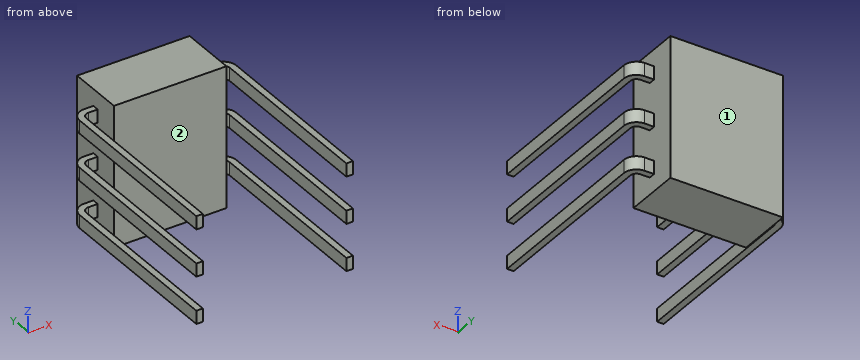
Autodesk Inventor part; units mm, degrees
ref_plane "YZ Plane" through (0, 0, 0) normal (1, 0, 0) x (0, 1, 0)
ref_plane "XZ Plane" through (0, 0, 0) normal (0, 1, 0) x (-1, 0, 0)
ref_plane "XY Plane" through (0, 0, 0) normal (0, 0, 1) x (1, 0, 0)
sketch "Sketch2" plane through (0, 0, 0) normal (0, 0, 1) x (1, 0, 0)
  line L0 (3, -1.5) -> (-3, -1.5)
  line L1 (-3, -1.5) -> (-3, 1.5)
  line L2 (-3, 1.5) -> (3, 1.5)
  line L3 (3, 1.5) -> (3, -1.5)
  line L4 (3, -1.5) -> (-3, 1.5) construction
  line L5 (-3, -1.5) -> (3, 1.5) construction
  point P0 (0, 0)
  dimension "d4" = 6
  dimension "d5" = 3
extrude "Extrusion1" add sketch "Sketch2" along normal mid plane 7.5
ref_plane "Work Plane1" through (3, -1.5, 3.75) normal (1, 0, 0) x (0, 0, -1)
ref_plane "Work Plane4" through (0, 0, 2.5) normal (0, 0, 1) x (1, 0, 0)
ref_plane "Work Plane5" through (-3, -10, 3.75) normal (0, -1, 0) x (1, 0, 0)
sketch "Sketch25" plane through (0, 0, 2.5) normal (0, 0, 1) x (1, 0, 0)
  line L0 (3, -1.5) -> (3, 1.5)
  line L1 (3, 0) -> (3.5, 0)
  line L2 (4, -0.5) -> (4, -10)
  arc A0 (4, -0.5) -> (3.5, 0) centre (3.5, -0.5) ccw
  point P0 (0, 0)
  point P1 (4, 0)
  dimension "d44" = 1
  dimension "d45" = 10
  dimension "d46" = 0.5
sketch "Sketch26" plane through (-3, -10, 3.75) normal (0, -1, 0) x (1, 0, 0)
  line L0 (6.824, -0.8954) -> (7.174, -0.8954)
  line L1 (7.174, -0.8954) -> (7.174, -1.5954)
  line L2 (7.174, -1.5954) -> (6.824, -1.5954)
  line L3 (6.824, -1.5954) -> (6.824, -0.8954)
  line L4 (6.824, -0.8954) -> (7.174, -1.5954) construction
  line L5 (7.174, -0.8954) -> (6.824, -1.5954) construction
  point P0 (3, -3.75)
  point P1 (6.999, -1.2454)
  dimension "d37" = 0.35
  dimension "d38" = 0.7
sweep "Sweep2" add profiles "Sketch26" path "Sketch25" path curves L2 A0 L1
pattern_linear "Rectangular Pattern2" count 3 spacing 2.5 along (0, 0, -1) of "Sweep2"
mirror "Mirror2" about plane through (0, 0, 0) normal (1, 0, 0) of "Sweep2", "Rectangular Pattern2"
properties part number "DetalV2(legs)"
Design review of the part built by this model. Coordinates are the model's own, in mm. Face numbers are marked on the shaded views. A direction names the side the tool comes from. Coordinates: 2 decimals unless noted, no trailing zeros. Order: outer loops, then holes, each group sorted by start corner. A loop starts at its lowest first (then second) coordinate and runs counter-clockwise, first axis right, second up.
Item 1: Take a section at B-B, the plane z = -1.5. Write out the cut boundary in (x, y), then the cut area to 3 significant figures.
Item 2: For line 1 (Z direction, x = -3.5, y = 0); line 2 (X direction, y = -0.75, z = 2.25); line 3 (X direction, y = -6, z = -0.25), list the stretches that pass through material, from the lowest coordinate up.
Item 3: For the marked faces 1 and 2, list the 3-axis set-ups (+Z, -Z, +X, -X, +Y, -Y) from which the entire face can be reached by the end or side of a thin tool; tool diameter is ignored.
Item 4: Take a section at A-A, the plane y = -8.5. Write out the cut boundary in (x, z), then the cut area to 3 significant figures.
Item 5: Take a section at C-C, the plane y = 0.5. Write out the cut boundary in (x, z).
Item 6: For pin 1 Ø0.9 at (x, y) = (-3.5, -6.5) entering from -Z; pin 2 Ø2 at (x, z) = (-1.5, 0) entering from -Y; pin 3 Ø1 at (x, y) = (2.5, -8) entering from -Z; pin 4 Ø0.9 at (x, y) = (-3.5, -6.5) entering from +Z, all flat-tipped, find the tip position at first contact; note any pin that passes through.
The answers:
1. outline: (-3, -1.5) - (3, -1.5) - (3, 1.5) - (-3, 1.5) - close
1. area: 18.0 mm2
2. line 1: z = -2.85 to -2.15, -0.35 to 0.35, 2.15 to 2.85
2. line 2: x = -4.17 to -3.82, -3 to 3, 3.82 to 4.17
2. line 3: x = -4.17 to -3.82, 3.82 to 4.17
3. face 1: +Z, -Z, +X, -X, +Y
3. face 2: +Z, -Z, -Y
4. outline: (-4.17, -2.85) - (-3.82, -2.85) - (-3.82, -2.15) - (-4.17, -2.15) - close; (-4.17, -0.35) - (-3.82, -0.35) - (-3.82, 0.35) - (-4.17, 0.35) - close; (-4.17, 2.15) - (-3.82, 2.15) - (-3.82, 2.85) - (-4.17, 2.85) - close; (3.82, -2.85) - (4.17, -2.85) - (4.17, -2.15) - (3.82, -2.15) - close; (3.82, -0.35) - (4.17, -0.35) - (4.17, 0.35) - (3.82, 0.35) - close; (3.82, 2.15) - (4.17, 2.15) - (4.17, 2.85) - (3.82, 2.85) - close
4. area: 1.47 mm2
5. outline: (-3, -3.75) - (3, -3.75) - (3, 3.75) - (-3, 3.75) - close
6. pin 1: stops at z = -2.85
6. pin 2: stops at y = -1.5
6. pin 3: passes through
6. pin 4: stops at z = 2.85
